Geometry check sheet. Reference: the model listing, model coordinates, mm. Face numbers are marked on the shaded views. A direction names the side the tool comes from. Coordinates: 2 decimals unless noted, no trailing zeros. Write each loop counter-clockwise with the first axis right and the second up, starting at its lowest first coordinate (ties: lowest second). Pieces come first, ordered by that corner, then holes. Notation, with made-up numbers: (27, 45) -> (83, 45) arc R27 cw to (83, 76) -> close; hole circle Ø6 at (-35, -24.75). An arc over 180 degrees is marked (long way). Answer in a Markdown table with one row per item. Add a question column.
1. Depth check by flat-ended pin: P1, Ø4, axis at x = -6.5, y = 6, coming from the +Z side; P2, Ø5.5, axis at x = 0, y = 0, coming from the -Z side. Enter the tip coordinate at first touch or a pass-through.
2. Cross-section at D-D on x = -5. Record the cut outline in (y, z).
3. Cross-section at A-A on y = 0. Record the cut outline in (x, z), and give its area (3 significant figures).
4. Cross-section at C-C on z = 3.75. Record the cut outline in (x, y), and give its area (3 significant figures).
5. Set-up check for the marked faces 1 and 2: record each of +Z, -Z, +X, -X, +Y, -Y from which the full face is reachable in a straight line by a thin tool's end or side.
6. Mould release check, pull along Y, two halves, no side actions. Record for the marked faces 3, 4 and 5: pulls with the +Y half, pulls with the -Y half, needs draft (parallel to the pull), parting line crosses it, or undercut.
7. Cross-section at B-B on x = 0. Record the cut outline in (y, z).
8. Scan lines: L1, parallel to Y at x = 8.25, z = 0.75; L2, parallel to Z at x = 2.5, y = 4; L3, parallel to Y at x = 0, z = -0.5. Record each from-to range of solid material in increasing order. Write a range as from..to.
```python
from build123d import *

# Parameters (mm, degrees)
SKETCH1_R                  = 1.75
BASE_FLANGE1_DEPTH         = 2
SKETCHED_START             = -24
SKETCHED_BEND1_OUTLINE_W   = 20
SKETCHED_BEND1_OUTLINE_H   = 2
SKETCHED_BEND1_DEPTH       = 12.627322451
SKETCHED_START_2           = 11.372677549
SKETCHED_BEND1_2_OUTLINE_W = 20
SKETCHED_BEND1_2_OUTLINE_H = 2
SKETCHED_BEND1_2_DEPTH     = 12.627322451
SKETCHED_START_3           = -11.114397241
SKETCHED_BEND1_3_DEPTH     = 1.741719692
SKETCHED_START_4           = 9.372677549
SKETCHED_BEND1_4_DEPTH     = 1.710960308
SKETCHED_START_5           = 8.636077549
SKETCHED_BEND1_5_DEPTH     = 2.7366
SKETCHED_START_6           = -11.372677549
SKETCHED_BEND1_6_DEPTH     = 2.7366
SKETCHED_START_7           = -10
SKETCHED_BEND1_7_DEPTH     = 20


with BuildPart() as part:
    # Base-Flange1: sheet metal written as solids
    # Sketch1 → Base-Flange1 (new body)
    with BuildSketch(Plane.XY):
        with BuildLine():
            Line((-10, 23.376973739), (-10, -23.376973739))
            ThreePointArc((-10, -23.376973739), (0, -22), (10, -23.376973739))
            Line((10, -23.376973739), (10, 23.376973739))
            ThreePointArc((10, 23.376973739), (0, 22), (-10, 23.376973739))
        make_face()
        Circle(SKETCH1_R, mode=Mode.SUBTRACT)
    extrude(amount=-BASE_FLANGE1_DEPTH)

    # Sketched Bend1: read off the stored shape, not the designer's step
    # Sketched Bend1 outline → Sketched Bend1 (cut)
    with BuildSketch(Plane(origin=(0, 0, 0), x_dir=(1, 0, 0), z_dir=(0, 1, 0)).offset(SKETCHED_START)):
        with Locations((0, 1)):
            Rectangle(SKETCHED_BEND1_OUTLINE_W, SKETCHED_BEND1_OUTLINE_H)
    extrude(amount=SKETCHED_BEND1_DEPTH, mode=Mode.SUBTRACT)

    # Sketched Bend1 2 outline → Sketched Bend1 2 (cut)
    with BuildSketch(Plane(origin=(0, 0, 0), x_dir=(1, 0, 0), z_dir=(0, 1, 0)).offset(SKETCHED_START_2)):
        with Locations((0, 1)):
            Rectangle(SKETCHED_BEND1_2_OUTLINE_W, SKETCHED_BEND1_2_OUTLINE_H)
    extrude(amount=SKETCHED_BEND1_2_DEPTH, mode=Mode.SUBTRACT)

    # Sketched Bend1 3 outline → Sketched Bend1 3 (add)
    with BuildSketch(Plane(origin=(0, 0, 0), x_dir=(1, 0, 0), z_dir=(0, 1, 0)).offset(SKETCHED_START_3)):
        with BuildLine():
            Line((10, 0), (-10, 0))
            Line((-10, 0), (-10, -12.749651288))
            ThreePointArc((-10, -12.749651288), (0, -11.372677549), (10, -12.749651288))
            Line((10, -12.749651288), (10, 0))
        make_face()
    extrude(amount=SKETCHED_BEND1_3_DEPTH)

    # Sketched Bend1 4 outline → Sketched Bend1 4 (add)
    with BuildSketch(Plane(origin=(0, 0, 0), x_dir=(1, 0, 0), z_dir=(0, 1, 0)).offset(SKETCHED_START_4)):
        with BuildLine():
            Line((10, 0), (-10, 0))
            Line((-10, 0), (-10, -12.749651288))
            ThreePointArc((-10, -12.749651288), (0, -11.372677549), (10, -12.749651288))
            Line((10, -12.749651288), (10, 0))
        make_face()
    extrude(amount=SKETCHED_BEND1_4_DEPTH)

    # Sketched Bend1 5 outline → Sketched Bend1 5 (add)
    with BuildSketch(Plane(origin=(0, 0, 0), x_dir=(1, 0, 0), z_dir=(0, 1, 0)).offset(SKETCHED_START_5)):
        with BuildLine():
            Line((-10, 0), (-10, -12.749651288))
            ThreePointArc((-10, -12.749651288), (0, -11.372677549), (10, -12.749651288))
            Line((10, -12.749651288), (10, 0))
            Line((10, 0), (-10, 0))
        make_face()
    extrude(amount=SKETCHED_BEND1_5_DEPTH)

    # Sketched Bend1 6 outline → Sketched Bend1 6 (add)
    with BuildSketch(Plane(origin=(0, 0, 0), x_dir=(1, 0, 0), z_dir=(0, 1, 0)).offset(SKETCHED_START_6)):
        with BuildLine():
            Line((-10, 0), (-10, -12.749651288))
            ThreePointArc((-10, -12.749651288), (0, -11.372677549), (10, -12.749651288))
            Line((10, -12.749651288), (10, 0))
            Line((10, 0), (-10, 0))
        make_face()
    extrude(amount=SKETCHED_BEND1_6_DEPTH)

    # Sketched Bend1 7 outline → Sketched Bend1 7 (cut)
    with BuildSketch(Plane.YZ.offset(SKETCHED_START_7)):
        with BuildLine():
            Line((-11.372677549, -2), (-8.636077549, -2))
            ThreePointArc((-8.636077549, -2), (-10.571145966, -1.198468418), (-11.372677549, 0.7366))
            Line((-11.372677549, 0.7366), (-11.372677549, -2))
        make_face()
        with BuildLine():
            ThreePointArc((11.372677549, 0.7366), (10.571145966, -1.198468418), (8.636077549, -2))
            Line((8.636077549, -2), (11.372677549, -2))
            Line((11.372677549, -2), (11.372677549, 0.7366))
        make_face()
        with BuildLine():
            Line((-8.636077549, 14), (-9.372677549, 14))
            Line((-9.372677549, 14), (-9.372677549, 0.7366))
            ThreePointArc((-9.372677549, 0.7366), (-9.156932404, 0.215745145), (-8.636077549, 0))
            Line((-8.636077549, 0), (-8.636077549, 14))
        make_face()
        with BuildLine():
            Line((9.372677549, 0.7366), (9.372677549, 14))
            Line((9.372677549, 14), (8.636077549, 14))
            Line((8.636077549, 14), (8.636077549, 0))
            ThreePointArc((8.636077549, 0), (9.156932404, 0.215745145), (9.372677549, 0.7366))
        make_face()
    extrude(amount=SKETCHED_BEND1_7_DEPTH, mode=Mode.SUBTRACT)


solid = part.part
```
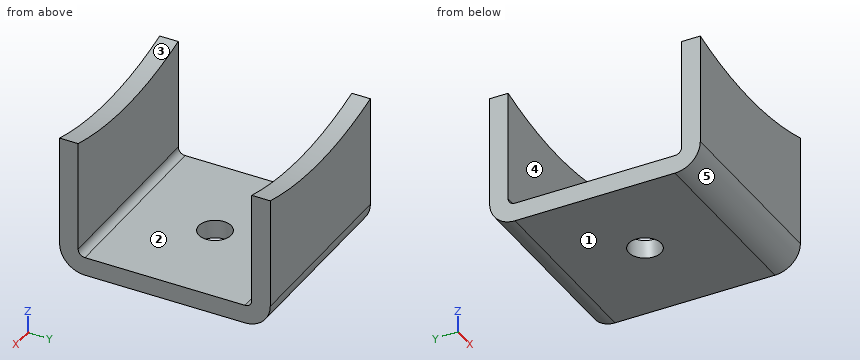
Results found:
| question | item | result |
|---|---|---|
| 1 | P1 | stops at z = 0 |
| 1 | P2 | stops at z = -2 |
| 2 | outline | (-11.37, 0.74) arc R2.74 ccw to (-8.64, -2) -> (8.64, -2) arc R2.74 ccw to (11.37, 0.74) -> (11.37, 11.71) -> (9.37, 11.71) -> (9.37, 0.74) arc R0.74 cw to (8.64, 0) -> (-8.64, 0) arc R0.74 cw to (-9.37, 0.74) -> (-9.37, 11.71) -> (-11.37, 11.71) -> close |
| 3 | outline | (-10, -2) -> (-1.75, -2) -> (-1.75, 0) -> (-10, 0) -> close; (1.75, -2) -> (10, -2) -> (10, 0) -> (1.75, 0) -> close |
| 3 | area | 33.0 mm^2 |
| 4 | outline | (-10, -11.37) -> (10, -11.37) -> (10, -9.37) -> (-10, -9.37) -> close; (-10, 9.37) -> (10, 9.37) -> (10, 11.37) -> (-10, 11.37) -> close |
| 4 | area | 80.0 mm^2 |
| 5 | face 1 | -Z, +X, -X, +Y, -Y |
| 5 | face 2 | +Z, +X, -X |
| 6 | face 3 | needs draft |
| 6 | face 4 | undercut |
| 6 | face 5 | pulls with the -Y half |
| 7 | outline | (-11.37, 0.74) arc R2.74 ccw to (-8.64, -2) -> (-1.75, -2) -> (-1.75, 0) -> (-8.64, 0) arc R0.74 cw to (-9.37, 0.74) -> (-9.37, 11.37) -> (-11.37, 11.37) -> close; (1.75, -2) -> (8.64, -2) arc R2.74 ccw to (11.37, 0.74) -> (11.37, 11.37) -> (9.37, 11.37) -> (9.37, 0.74) arc R0.74 cw to (8.64, 0) -> (1.75, 0) -> close |
| 8 | L1 | y = -11.37..-9.37, 9.37..11.37 |
| 8 | L2 | z = -2..0 |
| 8 | L3 | y = -11.08..-1.75, 1.75..11.08 |
